Verification items for the finished model (mm, model axes). A direction names the side the tool comes from. Round coordinates to 2 decimals unless told otherwise and drop trailing zeros. Write each loop counter-clockwise with the first axis right and the second up, starting at its lowest first coordinate (ties: lowest second). Pieces come first, ordered by that corner, then holes. Notation, with made-up numbers: (-36.75, 54.5) -> (-2.75, 54.5) arc R31 ccw to (-2.75, 81.5) -> close; hole circle Ø1 at (72.5, -35). An arc over 180 degrees is marked (long way). Answer as a JSON object with one key per item and string values. Group by question number.
(1) Draft check along X on faces 1 (the face through (0, -4, 2)), 2 (the face through (0, -3, -3)), 3 (the face through (6.5, 0.1, 0.5)), 4 (the face through (-3.5, -3, 0)). Enter one of: released by +X, released by -X, zero draft, split by the parting line, or undercut.
(2) Sectioned sample at A-A on y = -1.5. Record the cut outline in (x, z), and give its area (3 significant figures).
(3) Set-up check for faces 5 (the face through (-3, -4, -1)), 6 (the face through (6, 2, 0.25)), 7 (the face through (-2.801, 4.715, 1.644)), 8 (the face through (0, -3, 3)), 9 (the face through (3, 2, 0.25)): record each of +Z, -Z, +X, -X, +Y, -Y from which the full face is reachable in a straight line by a thin tool's end or side.
(4) Sectioned sample at D-D on y = -5.5. Record the cut outline in (x, z).
(5) Gauge pin test, flat ends, axial feed: pin 1 Ø3 at (x, z) = (5, -0.5) entering from -Y; pin 2 Ø2.5 at (x, z) = (0, 0) entering from +Y; pin 3 Ø1.3 at (y, z) = (-2, -0.5) entering from +X. Record the tip position at first contact, or that the pin passes through.
(6) Sectioned sample at B-B on x = -5.15. Record the cut outline in (y, z), and give its area (3 significant figures).
(7) Scan lines: L1, parallel to X at y = -1, z = 0.55; L2, parallel to X at y = 0, z = -1.55; L3, parallel to X at y = 0.25, z = 0.2. Record each from-to range of solid material in increasing order. Write a range as from..to.
```python
from build123d import *

# Parameters (mm, degrees)
BOSS_EXTRUDE1_DEPTH = 3
SKETCH4_W           = 0.5
SKETCH4_H           = 4
CUT_EXTRUDE2_DEPTH  = 13.56980509
SKETCH2_W           = 1
SKETCH2_H           = 0.5
CUT_EXTRUDE1_DEPTH  = 5.4
CUT_EXTRUDE3_DEPTH  = 1.5
SKETCH6_W           = 2.5
SKETCH6_H           = 5
CUT_EXTRUDE4_DEPTH  = 3
SKETCH7_R           = 0.2
BOSS_EXTRUDE2_DEPTH = 10.5


with BuildPart() as part:
    # Sketch1 → Boss-Extrude1 (new, symmetric)
    with BuildSketch(Plane.XY):
        with BuildLine():
            Line((-7, -5), (-7, 5))
            Line((-7, 5), (-3.5, 5))
            ThreePointArc((-3.5, 5), (-2.792893219, 4.707106781), (-2.5, 4))
            Line((-2.5, 4), (-2.5, -2.5))
            Line((-2.5, -2.5), (2.5, -2.5))
            Line((2.5, -2.5), (2.5, 4))
            ThreePointArc((2.5, 4), (2.792893219, 4.707106781), (3.5, 5))
            Line((3.5, 5), (7, 5))
            Line((7, 5), (7, -5))
            Line((7, -5), (-7, -5))
        make_face()
    extrude(amount=BOSS_EXTRUDE1_DEPTH, both=True)

    # Sketch4 → Cut-Extrude2 (cut, through all)
    with BuildSketch(Plane(origin=(0, 5, 0), x_dir=(1, 0, 0), z_dir=(0, 1, 0))):
        with Locations((-6.75, 0)):
            Rectangle(SKETCH4_W, SKETCH4_H)
        with Locations((6.75, 0)):
            Rectangle(SKETCH4_W, SKETCH4_H)
    extrude(amount=-CUT_EXTRUDE2_DEPTH, mode=Mode.SUBTRACT)

    # Sketch2 → Cut-Extrude1 (cut)
    with BuildSketch(Plane(origin=(0, 5, 0), x_dir=(1, 0, 0), z_dir=(0, 1, 0))):
        with Locations((-6, 0)):
            Rectangle(SKETCH2_W, SKETCH2_H)
        with Locations((-3, 0)):
            Rectangle(SKETCH2_W, SKETCH2_H)
        with Locations((3, 0)):
            Rectangle(SKETCH2_W, SKETCH2_H)
        with Locations((6, 0)):
            Rectangle(SKETCH2_W, SKETCH2_H)
    extrude(amount=-CUT_EXTRUDE1_DEPTH, mode=Mode.SUBTRACT)

    # Sketch5 → Cut-Extrude3 (cut)
    with BuildSketch(Plane.XZ.offset(5)):
        Polygon((-6, 2.5), (-3.5, 2.5), (-3.5, 1), (-2.5, 1), (-2.5, 2), (2.5, 2), (2.5, 1), (3.5, 1), (3.5, 2.5), (6, 2.5), (6, -2.5), (3.5, -2.5), (3.5, -1), (2.5, -1), (2.5, -2), (-2.5, -2), (-2.5, -1), (-3.5, -1), (-3.5, -2.5), (-6, -2.5), align=None)
    extrude(amount=-CUT_EXTRUDE3_DEPTH, mode=Mode.SUBTRACT)

    # Sketch6 → Cut-Extrude4 (cut)
    with BuildSketch(Plane.XZ.offset(3.5)):
        with Locations((-4.75, 0)):
            Rectangle(SKETCH6_W, SKETCH6_H)
        with Locations((4.75, 0)):
            Rectangle(SKETCH6_W, SKETCH6_H)
    extrude(amount=-CUT_EXTRUDE4_DEPTH, mode=Mode.SUBTRACT)

    # Sketch7 → Boss-Extrude2 (add)
    with BuildSketch(Plane.XZ.offset(0.5)):
        with Locations(Location((-5.15, -1.27, 0), (0, 0, 90))):
            Circle(SKETCH7_R)
        with Locations(Location((-5.15, 1.27, 0), (0, 0, 90))):
            Circle(SKETCH7_R)
        with Locations(Location((5.15, 1.27, 0), (0, 0, 90))):
            Circle(SKETCH7_R)
        with Locations(Location((5.15, -1.27, 0), (0, 0, 90))):
            Circle(SKETCH7_R)
    extrude(amount=BOSS_EXTRUDE2_DEPTH)


solid = part.part
```
Computed values:
{
 "1": {"face 1": "undercut", "face 2": "zero draft", "face 3": "released by +X", "face 4": "undercut"},
 "2": {"outline": "(-7, -3) -> (-2.5, -3) -> (-2.5, 3) -> (-7, 3) -> (-7, 2) -> (-6.5, 2) -> (-6.5, -2) -> (-7, -2) -> close; circle Ø0.4 at (-5.15, -1.27); circle Ø0.4 at (-5.15, 1.27); (2.5, -3) -> (7, -3) -> (7, -2) -> (6.5, -2) -> (6.5, 2) -> (7, 2) -> (7, 3) -> (2.5, 3) -> close; circle Ø0.4 at (5.15, -1.27); circle Ø0.4 at (5.15, 1.27); hole (-6, -2.5) -> (-3.5, -2.5) -> (-3.5, 2.5) -> (-6, 2.5) -> close; hole (3.5, -2.5) -> (6, -2.5) -> (6, 2.5) -> (3.5, 2.5) -> close", "area": "25.5 mm2"},
 "3": {"face 5": "-Y", "face 6": "+X, +Y", "face 7": "+Z, -Z, +Y", "face 8": "+Z, +X, -X, +Y, -Y", "face 9": "+Y"},
 "4": {"outline": "circle Ø0.4 at (-5.15, -1.27); circle Ø0.4 at (-5.15, 1.27); circle Ø0.4 at (5.15, -1.27); circle Ø0.4 at (5.15, 1.27)"},
 "5": {"pin 1": "y = -11", "pin 2": "y = -2.5", "pin 3": "x = 6.5"},
 "6": {"outline": "(-11, -1.47) -> (-0.5, -1.47) -> (-0.5, -2.5) -> (-5, -2.5) -> (-5, -3) -> (5, -3) -> (5, 3) -> (-5, 3) -> (-5, 2.5) -> (-0.5, 2.5) -> (-0.5, 1.47) -> (-11, 1.47) -> (-11, 1.07) -> (-0.5, 1.07) -> (-0.5, -1.07) -> (-11, -1.07) -> close", "area": "45.9 mm2"},
 "7": {"L1": "-6.5..-6, -3.5..-2.5, 2.5..3.5, 6..6.5", "L2": "-6.5..-2.5, 2.5..6.5", "L3": "-5.5..-3.5, 3.5..5.5"}
}
